Geometry: see drawing. Coordinates: mm, zero at the bounding-box minimum. A direction names the side the tool comes from. Coordinates: 2 decimals unless noted, no trailing zeros. Write each loop counter-clockwise with the first axis right and the second up, starting at its lowest first coordinate (ties: lowest second). Pieces come first, ordered by that corner, then holes. Notation, with made-up numbers: (62.25, 54.5) - (116.25, 54.5) arc R16 ccw to (116.25, 80.5) - close; hole circle Ø6 at (10, 1.5). An arc over 180 degrees is marked (long way). Use a Markdown table: item, result. Add a question column.
Q1. Section query C-C (x = 1.25). Return the cut outline in (y, z) (1 decimal).
Q2. Section query B-B (y = 2.75). Return the cut outline in (x, z) (1 decimal), then the cut area to 3 significant figures.
Q3. Set-up query: the marked faces 1 and 2. Return all of +Z, -Z, +X, -X, +Y, -Y with unobstructed straight access to the full face (end or side cutting, diameter ignored); none if empty.
Q4. Material intervals for probe 1 along X at (y, z) = (2.5, 12); probe 2 along Y at (x, z) = (1, 9); probe 3 along Z at (x, y) = (5, 5), sorted ascending. Write a range as from..to.
Q5. Pin query (flat end, axial travel): P1, Ø1.4, axis at y = 1.5, z = 10, coming from the -X side (1 decimal); P2, Ø1.3, axis at x = 3, z = 14.5, coming from the +Y side; P3, Ø0.7, axis at y = 5, z = 12.5, coming from the +X side. Return the tip coordinate at first contact, or that it passes through.
Q6. Section query A-A (z = 15.5). Return the cut outline in (x, y).
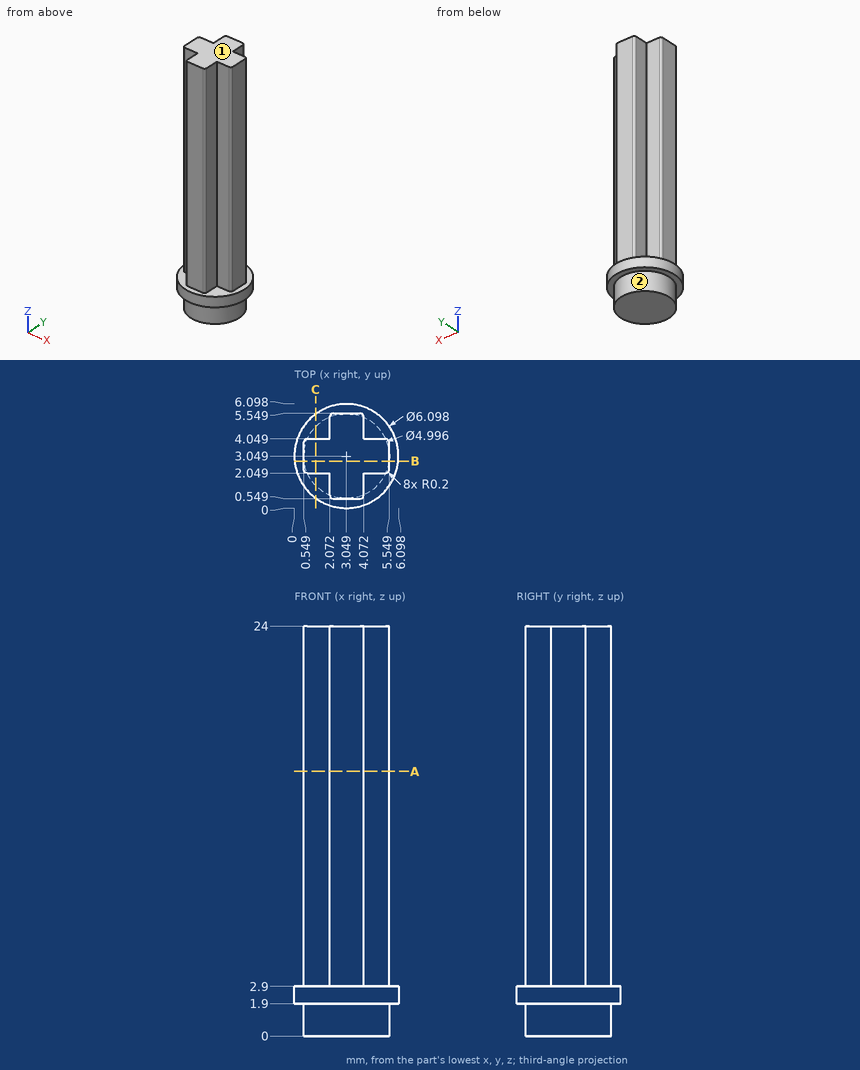
Values follow:
| question | item | result |
|---|---|---|
| 1 | outline | (0.6, 1.9) - (1.3, 1.9) - (1.3, 0) - (4.8, 0) - (4.8, 1.9) - (5.5, 1.9) - (5.5, 2.9) - (4, 2.9) - (4, 24) - (2, 24) - (2, 2.9) - (0.6, 2.9) - close |
| 2 | outline | (0, 1.9) - (0.6, 1.9) - (0.6, 0) - (5.5, 0) - (5.5, 1.9) - (6.1, 1.9) - (6.1, 2.9) - (5.5, 2.9) - (5.5, 24) - (0.5, 24) - (0.5, 2.9) - (0, 2.9) - close |
| 2 | area | 121 mm2 |
| 3 | face 1 | +Z, +X, -X, +Y, -Y |
| 3 | face 2 | -Z |
| 4 | probe 1 | 0.55..5.55 |
| 4 | probe 2 | 2.05..4.05 |
| 4 | probe 3 | 1.9..2.9 |
| 5 | P1 | x = 0.6 |
| 5 | P2 | y = 5.55 |
| 5 | P3 | x = 4.07 |
| 6 | outline | (0.55, 2.25) arc R0.2 ccw to (0.75, 2.05) - (2.07, 2.05) - (2.07, 0.75) arc R0.2 ccw to (2.27, 0.55) - (3.87, 0.55) arc R0.2 ccw to (4.07, 0.75) - (4.07, 2.05) - (5.35, 2.05) arc R0.2 ccw to (5.55, 2.25) - (5.55, 3.85) arc R0.2 ccw to (5.35, 4.05) - (4.07, 4.05) - (4.07, 5.35) arc R0.2 ccw to (3.87, 5.55) - (2.27, 5.55) arc R0.2 ccw to (2.07, 5.35) - (2.07, 4.05) - (0.75, 4.05) arc R0.2 ccw to (0.55, 3.85) - close |
